Answer from the drawing. Dimensions are ordinates in mm from the lowest x, y and z of the part. A direction names the side the tool comes from. Give positions to 0.01 mm unless a question says otherwise; leave off trailing zeros. Write each loop counter-clockwise with the first axis right and the second up, starting at its lowest first coordinate (ties: lowest second). Pieces come first, ordered by that corner, then holes. Notation, with made-up numbers: (-28.5, 41) - (22.5, 41) arc R20 cw to (22.5, 79) - close; hole circle Ø10 at (17.25, 40). An arc over 180 degrees is marked (long way). Write item = value, one per line.
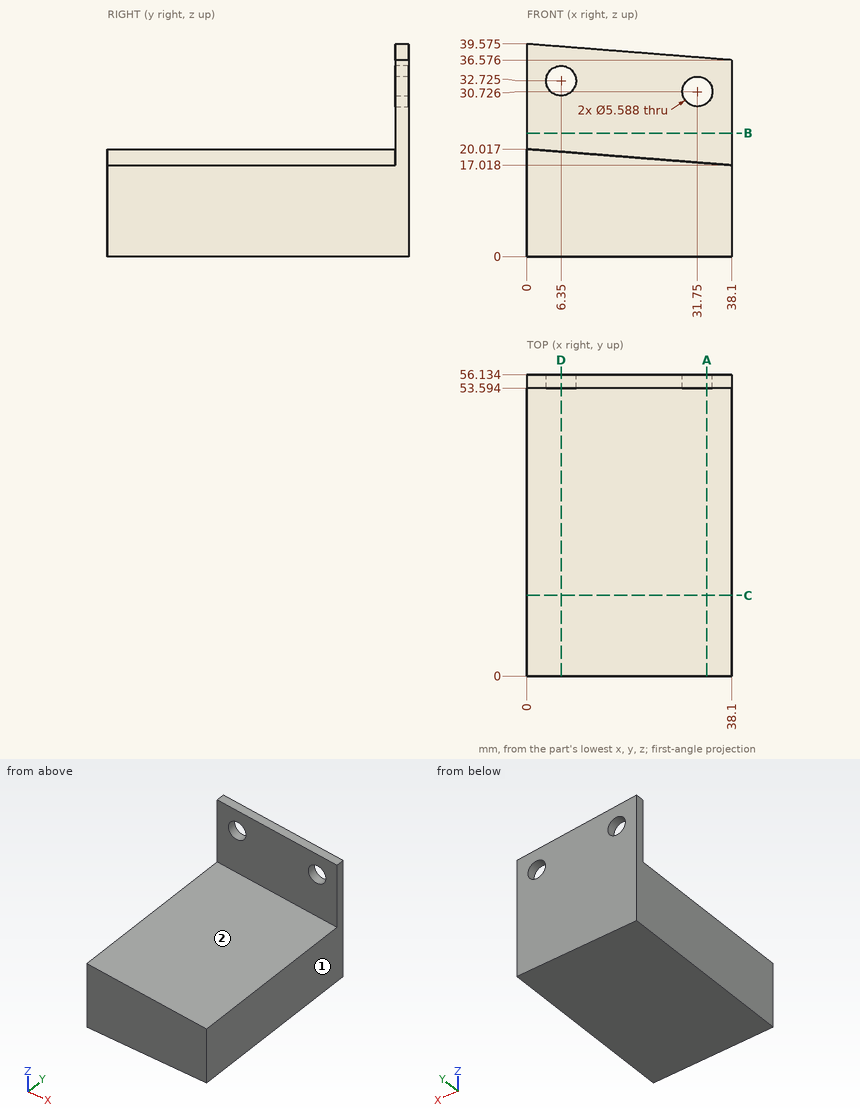
1. Find section A-A, the plane x = 33.5. Give the vertices of the cut face in (y, z), then the cut area to 3 significant figures.
Solution:
outline = (0, 0) - (56.13, 0) - (56.13, 28.55) - (53.59, 28.55) - (53.59, 17.38) - (0, 17.38) - close; (53.59, 32.9) - (56.13, 32.9) - (56.13, 36.94) - (53.59, 36.94) - close
area = 1,010 mm^2
2. Find section C-C, the plane y = 15. Give the vertices of the cut face in (x, z).
Solution:
outline = (0, 0) - (38.1, 0) - (38.1, 17.02) - (0, 20.02) - close
3. Find section D-D, the plane x = 6.35. Give the vertices of the cut face in (y, z) (1 decimal).
Solution:
outline = (0, 0) - (56.1, 0) - (56.1, 29.9) - (53.6, 29.9) - (53.6, 19.5) - (0, 19.5) - close; (53.6, 35.5) - (56.1, 35.5) - (56.1, 39.1) - (53.6, 39.1) - close
4. Straight lines are drawn through the part: line 1 (Z direction, x = 6, y = 54); line 2 (Y direction, x = 5.5, z = 28); line 3 (Z direction, x = 27, y = 12). For each, find the intervals that lie inside material, in ascending order.
Solution:
line_1 = 0 to 29.95, 35.5 to 39.1
line_2 = 53.59 to 56.13
line_3 = 0 to 17.89
5. Find section B-B, the plane z = 23. Give the vertices of the cut face in (x, y).
Solution:
outline = (0, 53.59) - (38.1, 53.59) - (38.1, 56.13) - (0, 56.13) - close
6. A tool of negligible diameter and unlimited length cuts with its end or side. For the marked faces 1 and 2, from which of +Z, -Z, +X, -X, +Y, -Y can it reach the whole face along a straight path? Write none if from no direction.
Solution:
face_1 = +Z, -Z, +X, +Y, -Y
face_2 = +Z, +X, -Y
7. Given pin 1 (7 mm diameter, centred on x = 18.5, z = 23.5, fed in from -Y); pin 2 (3 mm diameter, centred on x = 16, y = 23.5, fed in from -Z), each flat-ended and moving along its own axis, determine where each tip first touches the part or whether it passes through.
Solution:
pin_1 = 53.59
pin_2 = 0
